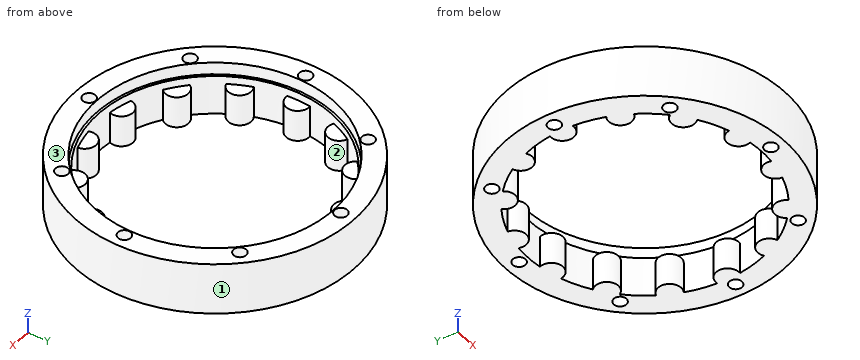
```python
from build123d import *

# Parameters (mm, degrees)
PINSBASEEXTRUDE_DEPTH      = 0.2
PINSBASEEXTRUDE_DEPTH_BACK = 0.2
PINSBASESKETCH_R           = 33
PINSEXTRUDE_START          = -0.2
PINSSKETCH_R               = 3
PINSEXTRUDE_DEPTH          = 8.6
PINSPATTERN_COUNT          = 14
BOREREVOLVESKETCH_W        = 4
BOREREVOLVESKETCH_H        = 7.5
SKETCH_4_R                 = 33
CUT_EXTRUDE_1_DEPTH        = 0.4
SKETCH_5_R                 = 36.5
SKETCH_5_R_2               = 30.5
EXTRUDE_3_DEPTH            = 13.5
CUT_EXTRUDE_2_REACH        = 55.355
SKETCH_6_R                 = 1.65
SKETCH_8_R                 = 31.1
CUT_EXTRUDE_3_DEPTH        = 3.2


with BuildPart() as part:
    # PinsBaseSketch → PinsBaseExtrude (new, two sides: drawn at the far end of the back side and taken through both)
    with BuildSketch(Plane.XY.offset(-PINSBASEEXTRUDE_DEPTH_BACK)):
        Circle(PINSBASESKETCH_R)
    extrude(amount=PINSBASEEXTRUDE_DEPTH + PINSBASEEXTRUDE_DEPTH_BACK)

    # PinsSketch → PinsExtrude (add)
    with BuildSketch(Plane.XY.offset(PINSEXTRUDE_START)):
        with Locations((30, 0)):
            Circle(PINSSKETCH_R)
    pinsextrude = extrude(amount=PINSEXTRUDE_DEPTH)

    # PinsPattern: PinsExtrude ×14 about axis
    pinspattern_axis = Axis((0, 0, 0), (0, 0, 1))
    for i in range(1, PINSPATTERN_COUNT):
        add(pinsextrude.rotate(pinspattern_axis, i * 360 / PINSPATTERN_COUNT))

    # BoreRevolveSketch → BoreRevolveCut (revolve, cut)
    with BuildSketch(Plane(origin=(0, 0, 0), x_dir=(0, 0, -1), z_dir=(1, 0, 0)), mode=Mode.PRIVATE) as borerevolvecut_sk:
        with Locations((0, 3.75)):
            Rectangle(BOREREVOLVESKETCH_W, BOREREVOLVESKETCH_H)
    revolve(borerevolvecut_sk.sketch.rotate(Axis((0, 0, 0), (0, 0, -1)), 90), axis=Axis((0, 0, 0), (0, 0, -1)), mode=Mode.SUBTRACT)

    # Sketch 4 → Cut-Extrude 1 (cut)
    with BuildSketch(Plane(origin=(0, 0, -0.2), x_dir=(-1, 0, 0), z_dir=(0, 0, -1))):
        Circle(SKETCH_4_R)
    extrude(amount=-CUT_EXTRUDE_1_DEPTH, mode=Mode.SUBTRACT)


with BuildPart() as cut_extrude_1_piece_1:
    # of the separate pieces the step leaves, piece 1, a body of its own (cut_extrude_1_pieces)
    add(part.part.solids().sort_by_distance((7.343190821, -32.172621102, 0.2))[0])



with BuildPart() as cut_extrude_1_piece_2:
    # of the separate pieces the step leaves, piece 2, a body of its own (cut_extrude_1_pieces)
    add(part.part.solids().sort_by_distance((20.575163461, -25.800438921, 0.2))[0])


with BuildPart() as cut_extrude_1_piece_3:
    # of the separate pieces the step leaves, piece 3, a body of its own (cut_extrude_1_pieces)
    add(part.part.solids().sort_by_distance((20.575163461, 25.800438921, 0.2))[0])


with BuildPart() as cut_extrude_1_piece_4:
    # of the separate pieces the step leaves, piece 4, a body of its own (cut_extrude_1_pieces)
    add(part.part.solids().sort_by_distance((-7.343190821, -32.172621102, 0.2))[0])


with BuildPart() as cut_extrude_1_piece_5:
    # of the separate pieces the step leaves, piece 5, a body of its own (cut_extrude_1_pieces)
    add(part.part.solids().sort_by_distance((29.731972641, -14.318163391, 0.2))[0])


with BuildPart() as cut_extrude_1_piece_6:
    # of the separate pieces the step leaves, piece 6, a body of its own (cut_extrude_1_pieces)
    add(part.part.solids().sort_by_distance((29.731972641, 14.318163391, 0.2))[0])


with BuildPart() as cut_extrude_1_piece_7:
    # of the separate pieces the step leaves, piece 7, a body of its own (cut_extrude_1_pieces)
    add(part.part.solids().sort_by_distance((-20.575163461, -25.800438921, 0.2))[0])


with BuildPart() as cut_extrude_1_piece_8:
    # of the separate pieces the step leaves, piece 8, a body of its own (cut_extrude_1_pieces)
    add(part.part.solids().sort_by_distance((-29.731972641, 14.318163391, 0.2))[0])


with BuildPart() as cut_extrude_1_piece_9:
    # of the separate pieces the step leaves, piece 9, a body of its own (cut_extrude_1_pieces)
    add(part.part.solids().sort_by_distance((-20.575163461, 25.800438921, 0.2))[0])


with BuildPart() as cut_extrude_1_piece_10:
    # of the separate pieces the step leaves, piece 10, a body of its own (cut_extrude_1_pieces)
    add(part.part.solids().sort_by_distance((33, 0, 0.2))[0])


with BuildPart() as cut_extrude_1_piece_11:
    # of the separate pieces the step leaves, piece 11, a body of its own (cut_extrude_1_pieces)
    add(part.part.solids().sort_by_distance((7.343190821, 32.172621102, 0.2))[0])


with BuildPart() as cut_extrude_1_piece_12:
    # of the separate pieces the step leaves, piece 12, a body of its own (cut_extrude_1_pieces)
    add(part.part.solids().sort_by_distance((-33, 0, 0.2))[0])


with BuildPart() as cut_extrude_1_piece_13:
    # of the separate pieces the step leaves, piece 13, a body of its own (cut_extrude_1_pieces)
    add(part.part.solids().sort_by_distance((-7.343190821, 32.172621102, 0.2))[0])


with BuildPart() as cut_extrude_1_piece_14:
    # of the separate pieces the step leaves, piece 14, a body of its own (cut_extrude_1_pieces)
    add(part.part.solids().sort_by_distance((-29.731972641, -14.318163391, 0.2))[0])


with BuildPart() as cut_extrude_1_piece_1_1:
    add(cut_extrude_1_piece_1.part)

    add(cut_extrude_1_piece_2.part)  # Extrude 3 merges Cut-Extrude 1 piece 2

    add(cut_extrude_1_piece_3.part)  # Extrude 3 merges Cut-Extrude 1 piece 3

    add(cut_extrude_1_piece_4.part)  # Extrude 3 merges Cut-Extrude 1 piece 4

    add(cut_extrude_1_piece_5.part)  # Extrude 3 merges Cut-Extrude 1 piece 5

    add(cut_extrude_1_piece_6.part)  # Extrude 3 merges Cut-Extrude 1 piece 6

    add(cut_extrude_1_piece_7.part)  # Extrude 3 merges Cut-Extrude 1 piece 7

    add(cut_extrude_1_piece_8.part)  # Extrude 3 merges Cut-Extrude 1 piece 8

    add(cut_extrude_1_piece_9.part)  # Extrude 3 merges Cut-Extrude 1 piece 9

    add(cut_extrude_1_piece_10.part)  # Extrude 3 merges Cut-Extrude 1 piece 10

    add(cut_extrude_1_piece_11.part)  # Extrude 3 merges Cut-Extrude 1 piece 11

    add(cut_extrude_1_piece_12.part)  # Extrude 3 merges Cut-Extrude 1 piece 12

    add(cut_extrude_1_piece_13.part)  # Extrude 3 merges Cut-Extrude 1 piece 13

    add(cut_extrude_1_piece_14.part)  # Extrude 3 merges Cut-Extrude 1 piece 14
    # Sketch 5 → Extrude 3 (add)
    with BuildSketch(Plane(origin=(0, 0, 0.2), x_dir=(-1, 0, 0), z_dir=(0, 0, -1))):
        Circle(SKETCH_5_R)
        Circle(SKETCH_5_R_2, mode=Mode.SUBTRACT)
    extrude(amount=-EXTRUDE_3_DEPTH)

    # Sketch 6 → Cut-Extrude 2 (cut, up to next)
    with BuildSketch(Plane.XY.offset(13.7), mode=Mode.PRIVATE) as cut_extrude_2_sk1:
        with Locations((-23.263814359, 23.263814295)):
            Circle(SKETCH_6_R)
    cut_extrude_2_tool1 = extrude(cut_extrude_2_sk1.sketch, amount=-CUT_EXTRUDE_2_REACH, mode=Mode.PRIVATE) & cut_extrude_1_piece_1_1.part
    # Sketch 6 → Cut-Extrude 2 (cut, up to next)
    with BuildSketch(Plane.XY.offset(13.7), mode=Mode.PRIVATE) as cut_extrude_2_sk2:
        with Locations((23.263811843, 23.263814295)):
            Circle(SKETCH_6_R)
    cut_extrude_2_tool2 = extrude(cut_extrude_2_sk2.sketch, amount=-CUT_EXTRUDE_2_REACH, mode=Mode.PRIVATE) & cut_extrude_1_piece_1_1.part
    # Sketch 6 → Cut-Extrude 2 (cut, up to next)
    with BuildSketch(Plane.XY.offset(13.7), mode=Mode.PRIVATE) as cut_extrude_2_sk3:
        with Locations((32.899998742, 1.194e-06)):
            Circle(SKETCH_6_R)
    cut_extrude_2_tool3 = extrude(cut_extrude_2_sk3.sketch, amount=-CUT_EXTRUDE_2_REACH, mode=Mode.PRIVATE) & cut_extrude_1_piece_1_1.part
    # Sketch 6 → Cut-Extrude 2 (cut, up to next)
    with BuildSketch(Plane.XY.offset(13.7), mode=Mode.PRIVATE) as cut_extrude_2_sk4:
        with Locations((23.263811843, -23.263811907)):
            Circle(SKETCH_6_R)
    cut_extrude_2_tool4 = extrude(cut_extrude_2_sk4.sketch, amount=-CUT_EXTRUDE_2_REACH, mode=Mode.PRIVATE) & cut_extrude_1_piece_1_1.part
    # Sketch 6 → Cut-Extrude 2 (cut, up to next)
    with BuildSketch(Plane.XY.offset(13.7), mode=Mode.PRIVATE) as cut_extrude_2_sk5:
        with Locations((-1.258e-06, -32.899998806)):
            Circle(SKETCH_6_R)
    cut_extrude_2_tool5 = extrude(cut_extrude_2_sk5.sketch, amount=-CUT_EXTRUDE_2_REACH, mode=Mode.PRIVATE) & cut_extrude_1_piece_1_1.part
    # Sketch 6 → Cut-Extrude 2 (cut, up to next)
    with BuildSketch(Plane.XY.offset(13.7), mode=Mode.PRIVATE) as cut_extrude_2_sk6:
        with Locations((-1.258e-06, 32.900001194)):
            Circle(SKETCH_6_R)
    cut_extrude_2_tool6 = extrude(cut_extrude_2_sk6.sketch, amount=-CUT_EXTRUDE_2_REACH, mode=Mode.PRIVATE) & cut_extrude_1_piece_1_1.part
    # Sketch 6 → Cut-Extrude 2 (cut, up to next)
    with BuildSketch(Plane.XY.offset(13.7), mode=Mode.PRIVATE) as cut_extrude_2_sk7:
        with Locations((-32.900001258, 1.194e-06)):
            Circle(SKETCH_6_R)
    cut_extrude_2_tool7 = extrude(cut_extrude_2_sk7.sketch, amount=-CUT_EXTRUDE_2_REACH, mode=Mode.PRIVATE) & cut_extrude_1_piece_1_1.part
    # Sketch 6 → Cut-Extrude 2 (cut, up to next)
    with BuildSketch(Plane.XY.offset(13.7), mode=Mode.PRIVATE) as cut_extrude_2_sk8:
        with Locations((-23.263814359, -23.263811907)):
            Circle(SKETCH_6_R)
    cut_extrude_2_tool8 = extrude(cut_extrude_2_sk8.sketch, amount=-CUT_EXTRUDE_2_REACH, mode=Mode.PRIVATE) & cut_extrude_1_piece_1_1.part
    add(cut_extrude_2_tool1.solids().sort_by_distance((-23.263814, 23.263814, 13.7))[0], mode=Mode.SUBTRACT)
    add(cut_extrude_2_tool2.solids().sort_by_distance((23.263812, 23.263814, 13.7))[0], mode=Mode.SUBTRACT)
    add(cut_extrude_2_tool3.solids().sort_by_distance((32.899999, 1e-06, 13.7))[0], mode=Mode.SUBTRACT)
    add(cut_extrude_2_tool4.solids().sort_by_distance((23.263812, -23.263812, 13.7))[0], mode=Mode.SUBTRACT)
    add(cut_extrude_2_tool5.solids().sort_by_distance((-1e-06, -32.899999, 13.7))[0], mode=Mode.SUBTRACT)
    add(cut_extrude_2_tool6.solids().sort_by_distance((-1e-06, 32.900001, 13.7))[0], mode=Mode.SUBTRACT)
    add(cut_extrude_2_tool7.solids().sort_by_distance((-32.900001, 1e-06, 13.7))[0], mode=Mode.SUBTRACT)
    add(cut_extrude_2_tool8.solids().sort_by_distance((-23.263814, -23.263812, 13.7))[0], mode=Mode.SUBTRACT)

    # Sketch 8 → Cut-Extrude 3 (cut)
    with BuildSketch(Plane.XY.offset(13.7)):
        with Locations((-1.258e-06, 1.194e-06)):
            Circle(SKETCH_8_R)
    extrude(amount=-CUT_EXTRUDE_3_DEPTH, mode=Mode.SUBTRACT)


solid = cut_extrude_1_piece_1_1.part
```
Design review of the part built by this model. Coordinates are the model's own, in mm. Face numbers are marked on the shaded views. Round coordinates to 2 decimals unless told otherwise and drop trailing zeros.
Item 1: For probe 1 along X at (y, z) = (21.5, 6.25); probe 2 along Y at (x, z) = (-16, 7.75); probe 3 along Y at (x, z) = (-24.5, 11.75), list the stretches that pass through material, from the lowest coordinate up.
Item 2: Clearance check with flat-ended pins moving along their axes: pin 1 Ø1.2 at (x, y) = (6, 29) entering from +Z; pin 2 Ø2 at (x, y) = (23.26, -23.26) entering from +Z; pin 3 Ø2.5 at (x, y) = (-26, 14) entering from +Z; pin 4 Ø1.5 at (y, z) = (-23.5, 6) entering from -X. State where each tip first meets the part, or that it passes through.
Item 3: We need section A-A on z = 9.5. State how many separate pieces and enclosed holes the cut face has, and give its area (3 significant figures).
Item 4: The part is to be moulded in two halves that separate along Y. For the marked faces 1, 2 and 3, say which applies: +Y half, -Y half, draft (parallel to the pull), parting line (faces both ways), or undercut.
Returned:
1. probe 1: x = -29.5 to -21.63, -20.98 to -16.43, 16.43 to 20.98, 21.63 to 29.5
1. probe 2: y = -32.81 to -25.97, -24.75 to -22.16, 22.16 to 24.75, 25.97 to 32.81
1. probe 3: y = -27.06 to -24.36, -22.17 to -19.16, 19.16 to 22.17, 24.36 to 27.06
2. pin 1: stops at z = 8.4
2. pin 2: passes through
2. pin 3: stops at z = 10.5
2. pin 4: stops at x = -28.54
3. separate pieces: 1
3. enclosed holes: 9
3. area: 1,190 mm2
4. face 1: parting line
4. face 2: undercut
4. face 3: draft
